Drawing for the job (mm, zero at the part's lowest x, y, z). Round coordinates to 2 decimals unless told otherwise and drop trailing zeros. Loops run counter-clockwise (first coordinate to the right, second up) from the corner with the lowest first, then second, coordinate; pieces in that order, holes last. Notation, with made-up numbers: M -18.75,56 L 3.25,56 A19 cw 3.25,79 Z; hole C 60.25,75.5 d5. An arc over 180 degrees is marked long. Answer in a Markdown table with one row per item.
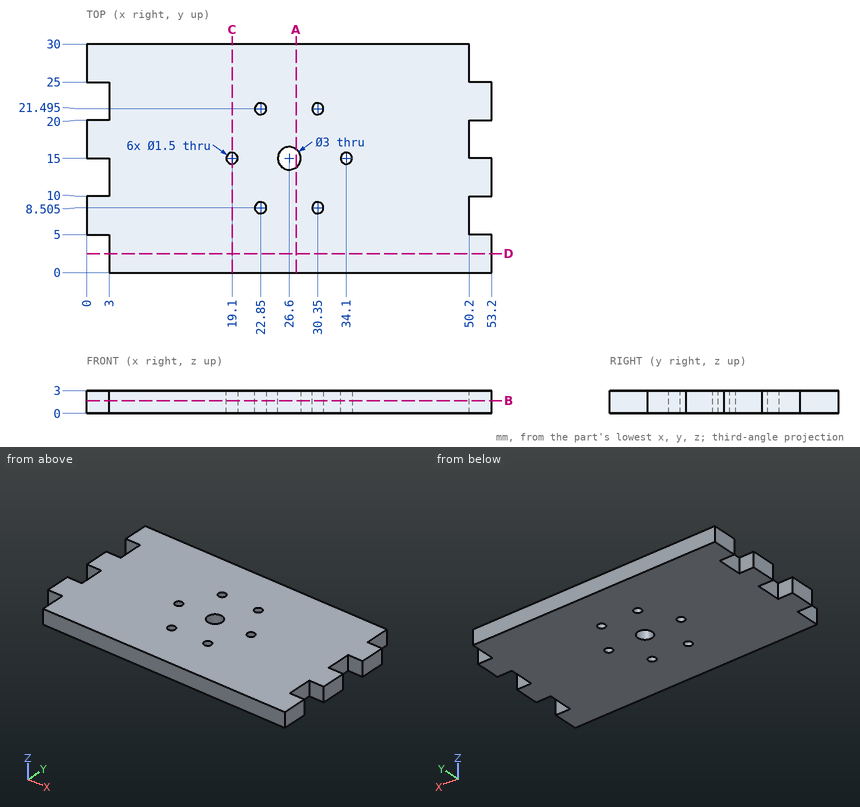
1. Saw through at A-A (x = 27.5). Write the cut outline in (y, z).
Verdict:
| item | result |
|---|---|
| outline | M 0,0 L 13.8,0 L 13.8,3 L 0,3 Z; M 16.2,0 L 30,0 L 30,3 L 16.2,3 Z |
2. Saw through at C-C (x = 19.1). Write the cut outline in (y, z), and give its area (3 significant figures).
Verdict:
| item | result |
|---|---|
| outline | M 0,0 L 14.25,0 L 14.25,3 L 0,3 Z; M 15.75,0 L 30,0 L 30,3 L 15.75,3 Z |
| area | 85.5 mm² |
3. Pin check, flat tips, straight feed: pin 1 (0.9 mm diameter, centred on x = 22.85, y = 21.5, fed in from +Z); pin 2 (0.9 mm diameter, centred on y = 12.5, z = 1, fed in from -X); pin 3 (1.5 mm diameter, centred on x = 51.5, z = 1.5, fed in from -Y); pin 4 (1.5 mm diameter, centred on y = 16.5, z = 1.5, fed in from +X). Stop position of each tip, or through.
Verdict:
| item | result |
|---|---|
| pin 1 | passes through |
| pin 2 | stops at x = 3 |
| pin 3 | stops at y = 0 |
| pin 4 | stops at x = 50.2 |
4. Saw through at B-B (z = 1.7). State how many separate pieces and enclosed holes the cut face has, and give its area (3 significant figures).
Verdict:
| item | result |
|---|---|
| separate pieces | 1 |
| enclosed holes | 7 |
| area | 1,490 mm² |
5. Wall check: probe 1 along Y at (x, z) = (34.1, 2.2); probe 2 along Y at (x, z) = (30.35, 1.25) (1 decimal); probe 3 along X at (y, z) = (1.5, 1.5). Give the ranges that are in metal, low to high.
Verdict:
| item | result |
|---|---|
| probe 1 | y = 0 to 14.25, 15.75 to 30 |
| probe 2 | y = 0 to 7.8, 9.3 to 20.7, 22.2 to 30 |
| probe 3 | x = 3 to 53.2 |
6. Saw through at D-D (y = 2.5). Write the cut outline in (x, z).
Verdict:
| item | result |
|---|---|
| outline | M 3,0 L 53.2,0 L 53.2,3 L 3,3 Z |
